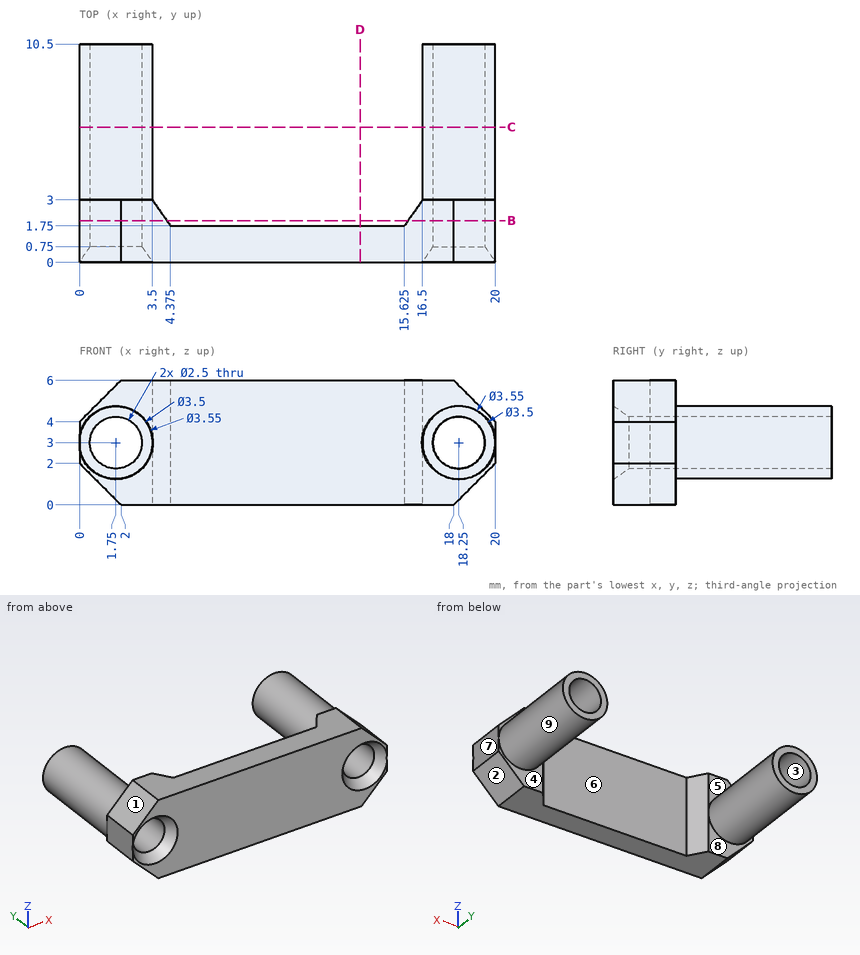
For this review, use the dimensioned drawing (mm, ordinates from the lowest corner) and the shaded views. A direction names the side the tool comes from. Round coordinates to 2 decimals unless told otherwise and drop trailing zeros. Order: outer loops, then holes, each group sorted by start corner. A loop starts at its lowest first (then second) coordinate and runs counter-clockwise, first axis right, second up. Notation, with made-up numbers: M -33,86.5 L 7,86.5 A22 cw 7,97.5 Z; hole C -30,38 d3. An arc over 180 degrees is marked long. Use a Markdown table: item, result.
1) Tool access review of the marked faces 5, 6, 7, 8 and 9: name each direction out of +Z, -Z, +X, -X, +Y, -Y from which nothing blocks a thin tool from reaching the whole face with its end or side.
Report:
| item | result |
|---|---|
| face 5 | +Z, +Y |
| face 6 | +Z, -Z, +Y |
| face 7 | +Z, -Z, +X, +Y, -Y |
| face 8 | -Z, +Y |
| face 9 | +Y |
2) Wall thickness on line 1 along X through (y, z) = (1.2, 3); line 2 along X through (y, z) = (4, 2.5) (1 decimal); line 3 along Y through (x, z) = (17, 5): over which ranges is each line inside the solid? List them lowest first. Write a range as [from, to].
Report:
| item | result |
|---|---|
| line 1 | [0, 0.5], [3, 17], [19.5, 20] |
| line 2 | [0.1, 0.6], [2.9, 3.4], [16.6, 17.1], [19.4, 19.9] |
| line 3 | [0, 3] |
3) Insertion check: pin 1 (1 mm diameter, centred on y = 4, z = 3.5, fed in from +X); pin 2 (3 mm diameter, centred on x = 13, z = 4.5, fed in from +Y); pin 3 (3 mm diameter, centred on x = 1.75, z = 3, fed in from -Y). Each pin has a flat end and moves straight along its axis. Give the tip position at first contact, or say it passes through.
Report:
| item | result |
|---|---|
| pin 1 | x = 20 |
| pin 2 | y = 1.75 |
| pin 3 | y = 0.39 |
4) Consider section C-C (y = 6.5). Write out the cut boundary in (x, z).
Report:
| item | result |
|---|---|
| outline | C 1.75,3 d3.5; C 18.25,3 d3.5; hole C 1.75,3 d2.5; hole C 18.25,3 d2.5 |
5) Draft analysis for pull direction X (two halves, no side actions). For the marked faces 1, 2, 3 and 4, state which applies: released by +X, released by -X, zero draft, split by the parting line, or undercut.
Report:
| item | result |
|---|---|
| face 1 | released by -X |
| face 2 | released by +X |
| face 3 | undercut |
| face 4 | undercut |
6) Consider section B-B (y = 2). Write out the cut boundary in (x, z).
Report:
| item | result |
|---|---|
| outline | M 0,2 L 2,0 L 4.2,0 L 4.2,6 L 2,6 L 0,4 Z; M 15.8,0 L 18,0 L 20,2 L 20,4 L 18,6 L 15.8,6 Z; hole C 1.75,3 d2.5; hole C 18.25,3 d2.5 |
7) Consider section D-D (x = 13.5). Write out the cut boundary in (y, z), then the cut area to 3 significant figures.
Report:
| item | result |
|---|---|
| outline | M 0,0 L 1.75,0 L 1.75,6 L 0,6 Z |
| area | 10.5 mm^2 |
